from build123d import *

# Parameters (mm, degrees)
SKETCH_1_W          = 240
SKETCH_1_H          = 240
SKETCH_1_R          = 60
EXTRUDE_1_DEPTH     = 8
SKETCH_2_R          = 2.75
SKETCH_2_R_2        = 3.75
CUT_EXTRUDE_1_DEPTH = 10
FILLET_1_R          = 10
SKETCH_3_R          = 6
CUT_EXTRUDE_2_DEPTH = 5.5


with BuildPart() as part:
    # 草图1 → 凸台-拉伸1 (new body)
    with BuildSketch(Plane(origin=(0, 0, 0), x_dir=(1, 0, 0), z_dir=(0, 1, 0))):
        with Locations((120, -120)):
            Rectangle(SKETCH_1_W, SKETCH_1_H)
        with Locations(Location((120, -120, 0), (0, 0, 270))):
            Circle(SKETCH_1_R, mode=Mode.SUBTRACT)
    extrude(amount=EXTRUDE_1_DEPTH)

    # 草图2 → 切除-拉伸1 (cut)
    with BuildSketch(Plane(origin=(0, 8, 0), x_dir=(1, 0, 0), z_dir=(0, 1, 0))):
        with Locations(Location((92.293791985, -43.619841991, 0), (0, 0, 270))):
            Circle(SKETCH_2_R)
        with Locations(Location((147.706208015, -43.619841991, 0), (0, 0, 270))):
            Circle(SKETCH_2_R)
        with Locations(Location((172.294053173, -57.815641012, 0), (0, 0, 270))):
            Circle(SKETCH_2_R)
        with Locations(Location((182.184358988, -67.705946827, 0), (0, 0, 270))):
            Circle(SKETCH_2_R)
        with Locations(Location((196.380158009, -92.293791985, 0), (0, 0, 270))):
            Circle(SKETCH_2_R)
        with Locations(Location((196.380158009, -147.706208015, 0), (0, 0, 270))):
            Circle(SKETCH_2_R)
        with Locations(Location((182.184358988, -172.294053173, 0), (0, 0, 270))):
            Circle(SKETCH_2_R)
        with Locations(Location((172.294053173, -182.184358988, 0), (0, 0, 270))):
            Circle(SKETCH_2_R)
        with Locations(Location((147.706208015, -196.380158009, 0), (0, 0, 270))):
            Circle(SKETCH_2_R)
        with Locations(Location((92.293791985, -196.380158009, 0), (0, 0, 270))):
            Circle(SKETCH_2_R)
        with Locations(Location((67.705946827, -182.184358988, 0), (0, 0, 270))):
            Circle(SKETCH_2_R)
        with Locations(Location((57.815641012, -172.294053173, 0), (0, 0, 270))):
            Circle(SKETCH_2_R)
        with Locations(Location((43.619841991, -147.706208015, 0), (0, 0, 270))):
            Circle(SKETCH_2_R)
        with Locations(Location((43.619841991, -92.293791985, 0), (0, 0, 270))):
            Circle(SKETCH_2_R)
        with Locations(Location((57.815641012, -67.705946827, 0), (0, 0, 270))):
            Circle(SKETCH_2_R)
        with Locations(Location((67.705946827, -57.815641012, 0), (0, 0, 270))):
            Circle(SKETCH_2_R)
        with Locations(Location((220, -20, 0), (0, 0, 270))):
            Circle(SKETCH_2_R_2)
        with Locations(Location((20, -20, 0), (0, 0, 270))):
            Circle(SKETCH_2_R_2)
        with Locations(Location((20, -220, 0), (0, 0, 270))):
            Circle(SKETCH_2_R_2)
        with Locations(Location((220, -220, 0), (0, 0, 270))):
            Circle(SKETCH_2_R_2)
    extrude(amount=-CUT_EXTRUDE_1_DEPTH, mode=Mode.SUBTRACT)

    # 圆角1
    fillet_1_edges = [part.edges().sort_by_distance(p)[0] for p in [
        (0, 4, 0),
        (240, 4, 0),
        (240, 4, 240),
        (0, 4, 240),
    ]]
    fillet(fillet_1_edges, radius=FILLET_1_R)

    # 草图3 → 切除-拉伸2 (cut)
    with BuildSketch(Plane.XZ):
        with Locations(Location((147.706208015, 196.380158009, 0), (0, 0, 270))):
            Circle(SKETCH_3_R)
        with Locations(Location((172.294053173, 182.184358988, 0), (0, 0, 270))):
            Circle(SKETCH_3_R)
        with Locations(Location((182.184358988, 172.294053173, 0), (0, 0, 270))):
            Circle(SKETCH_3_R)
        with Locations(Location((196.380158009, 147.706208015, 0), (0, 0, 270))):
            Circle(SKETCH_3_R)
        with Locations(Location((196.380158009, 92.293791985, 0), (0, 0, 270))):
            Circle(SKETCH_3_R)
        with Locations(Location((182.184358988, 67.705946827, 0), (0, 0, 270))):
            Circle(SKETCH_3_R)
        with Locations(Location((172.294053173, 57.815641012, 0), (0, 0, 270))):
            Circle(SKETCH_3_R)
        with Locations(Location((147.706208015, 43.619841991, 0), (0, 0, 270))):
            Circle(SKETCH_3_R)
        with Locations(Location((92.293791985, 43.619841991, 0), (0, 0, 270))):
            Circle(SKETCH_3_R)
        with Locations(Location((67.705946827, 57.815641012, 0), (0, 0, 270))):
            Circle(SKETCH_3_R)
        with Locations(Location((57.815641012, 67.705946827, 0), (0, 0, 270))):
            Circle(SKETCH_3_R)
        with Locations(Location((43.619841991, 92.293791985, 0), (0, 0, 270))):
            Circle(SKETCH_3_R)
        with Locations(Location((43.619841991, 147.706208015, 0), (0, 0, 270))):
            Circle(SKETCH_3_R)
        with Locations(Location((57.815641012, 172.294053173, 0), (0, 0, 270))):
            Circle(SKETCH_3_R)
        with Locations(Location((67.705946827, 182.184358988, 0), (0, 0, 270))):
            Circle(SKETCH_3_R)
        with Locations(Location((92.293791985, 196.380158009, 0), (0, 0, 270))):
            Circle(SKETCH_3_R)
    extrude(amount=-CUT_EXTRUDE_2_DEPTH, mode=Mode.SUBTRACT)


solid = part.part
Work out the finished part from the listing and answer in its coordinate system (mm). A direction names the side the tool comes from. Give positions to 0.01 mm unless a question says otherwise; leave off trailing zeros. Loops run counter-clockwise (first coordinate to the right, second up) from the corner with the lowest first, then second, coordinate; pieces in that order, holes last. Notation, with made-up numbers: (7, 84.5) - (51, 84.5) arc R27 cw to (51, 109.5) - close; hole circle Ø8 at (21, 46). An arc over 180 degrees is marked (long way). Answer in a Markdown table with one row per item. Add a question column.
Q1. Each of these flat-tipped pins is pushed along its axis until it touches: P1, Ø13, axis at x = 182, z = 69.5, coming from the -Y side; P2, Ø11, axis at x = 172.29, z = 57.82, coming from the -Y side; P3, Ø3.5, axis at x = 196.38, z = 92.29, coming from the +Y side. Where does it stop, or does it pass through?
Q2. Consider line 1 along Z through (x, y) = (70.5, 1.75); line 2 along Z through (x, y) = (149, 7); line 3 along X through (y, z) = (2.25, 18.5). Determine where each line is inside the solid, lowest interval first.
Q3. A tool of negligible diameter and unlimited length cuts with its end or side. For faces 3 (the cylindrical face through (92.558, 2.712, 202.374)), 4 (the cylindrical face through (198.7, 6.77, 149.18)), from which of +Z, -Z, +X, -X, +Y, -Y can it reach the whole face along a straight path? Write none if from no direction.
Q4. Determine the mould class of faces 1 (the flat face through (65, 8, 92)), 2 (the cylindrical face through (170.59, 3.94, 152.26)) for opening direction Z: released by +Z, released by -Z, zero draft, split by the parting line, or undercut.
Q5. The part is cut by section A-A (z = 120). Determine the outline of the cut face in (x, y).
Q6. The part is cut by section C-C (z = 220). Determine the outline of the cut face in (x, y).
Q7. The part is cut by section D-D (x = 120). Determine the outline of the cut face in (y, z), and give its area (3 significant figures).
Q8. The part is cut by section B-B (x = 220). Determine the outline of the cut face in (y, z), and give its area (3 significant figures).
Solution:
| question | item | result |
|---|---|---|
| 1 | P1 | stops at y = 0 |
| 1 | P2 | stops at y = 5.5 |
| 1 | P3 | passes through |
| 2 | line 1 | z = 0 to 52.51, 63.13 to 86.09, 153.91 to 176.87, 187.49 to 240 |
| 2 | line 2 | z = 0 to 41.19, 46.05 to 67.47, 172.53 to 193.95, 198.81 to 240 |
| 2 | line 3 | x = 0 to 16.56, 23.44 to 216.56, 223.44 to 240 |
| 3 | face 3 | -Y |
| 3 | face 4 | +Y, -Y |
| 4 | face 1 | zero draft |
| 4 | face 2 | undercut |
| 5 | outline | (0, 0) - (60, 0) - (60, 8) - (0, 8) - close; (180, 0) - (240, 0) - (240, 8) - (180, 8) - close |
| 6 | outline | (0, 0) - (16.25, 0) - (16.25, 8) - (0, 8) - close; (23.75, 0) - (216.25, 0) - (216.25, 8) - (23.75, 8) - close; (223.75, 0) - (240, 0) - (240, 8) - (223.75, 8) - close |
| 7 | outline | (0, 0) - (8, 0) - (8, 60) - (0, 60) - close; (0, 180) - (8, 180) - (8, 240) - (0, 240) - close |
| 7 | area | 960 mm² |
| 8 | outline | (0, 0) - (8, 0) - (8, 16.25) - (0, 16.25) - close; (0, 23.75) - (8, 23.75) - (8, 216.25) - (0, 216.25) - close; (0, 223.75) - (8, 223.75) - (8, 240) - (0, 240) - close |
| 8 | area | 1,800 mm² |
